Autodesk Inventor part; units mm, degrees
ref_plane "YZ Plane" through (0, 0, 0) normal (1, 0, 0) x (0, 1, 0)
ref_plane "XZ Plane" through (0, 0, 0) normal (0, 1, 0) x (-1, 0, 0)
ref_plane "XY Plane" through (0, 0, 0) normal (0, 0, 1) x (1, 0, 0)
sketch "Skizze1" plane through (0, 0, 0) normal (0, 1, 0) x (-1, 0, 0)
  line L0 (0, 0) -> (30, 0)
  line L1 (30, 0) -> (30, 30)
  line L2 (30, 30) -> (0, 30)
  line L3 (0, 30) -> (0, 0)
  circle A0 centre (15, 15) radius 14.1
  dimension "d7" = 28.2
  dimension "d20" = 30
  dimension "d21" = 30
extrude "Extrusion1" add sketch "Skizze1" along normal blind 22 contours L3 L2 L1 L0 | A0
sketch "Skizze2" plane through (0, 22, 0) normal (0, 1, 0) x (1, 0, 0)
  line L0 (0, 0) -> (-30, 0)
  line L1 (-1.5, 0) -> (-28.5, 0)
  line L2 (-28.5, 0) -> (-28.5, -28.5)
  line L3 (-28.5, -28.5) -> (-1.5, -28.5)
  line L4 (-1.5, -28.5) -> (-1.5, 0)
  line L5 (-30, 0) -> (-30, -30)
  line L6 (0, -30) -> (0, 0)
  line L7 (-30, -30) -> (0, -30)
  dimension "d8" = 1.5
  dimension "d9" = 1.5
  dimension "d10" = 1.5
extrude "Extrusion2" cut sketch "Skizze2" against normal blind 22 contours L4 L3 L2 L0
sketch "Skizze5" plane through (0, 22, 0) normal (0, 1, 0) x (1, 0, 0)
  line L0 (-30, 0) -> (-30, -30)
  line L1 (0, 0) -> (-30, 0)
  line L2 (-30, 0) -> (-30, -30)
  line L3 (-30, -30) -> (0, -30)
  line L4 (0, -30) -> (0, 0)
  line L5 (-31.5556, 0) -> (-1.5, 0) construction
  circle A0 centre (-15, -15) radius 1.35
  line L6 (-1.5, -28.5) -> (-28.5, -28.5)
  line L7 (-1.5, 0) -> (-1.5, -28.5)
  line L8 (-28.5, -28.5) -> (-28.5, 0)
  line L9 (-1.5, -28.5) -> (-28.5, -28.5)
  dimension "d17" = 2.7
extrude "Extrusion4" add sketch "Skizze5" along normal blind 1.5
equation "\"Biegeradius\" = Stärke"
equation "\"BreiteBiegungsfreistellung\" = Stärke"
equation "\"TiefeBiegungsfreistellung\" = 0.5 * Stärke"
equation "\"GrößeEckenfreistellung\" = 4 * Stärke"
equation "\"MinimalRest\" = 2 * Stärke"
equation "\"Übergangsradius\" = Biegeradius"
equation "\"JacobiRadiusGröße\" = Biegeradius"
equation "\"Abstandsgröße\" = Stärke"
properties part number "Gehäuse Motor"
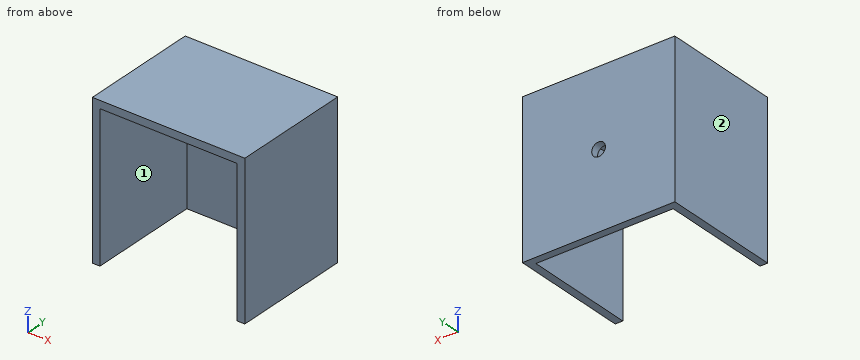
For this review, take the finished solid that the model builds, in its own axes (mm). Face numbers are marked on the shaded views. A direction names the side the tool comes from. Give positions to 0.01 mm unless a question says otherwise; leave off trailing zeros. Loops run counter-clockwise (first coordinate to the right, second up) from the corner with the lowest first, then second, coordinate; pieces in that order, holes last.
Item 1: Take a section at C-C, the plane x = -15.75. State the section outline as (y, z) points.
Item 2: Take a section at D-D, the plane x = -27.25. State the section outline as (y, z) points.
Item 3: Tool access review of the marked faces 1 and 2: name each direction out of +Z, -Z, +X, -X, +Y, -Y from which nothing blocks a thin tool from reaching the whole face with its end or side.
Item 4: Take a section at A-A, the plane z = 15. State the section outline as (x, y) points.
Item 5: Insertion check: pin 1 (2 mm diameter, centred on x = -23.5, z = 11.5, fed in from -Y); pin 2 (11 mm diameter, centred on x = -16, y = 8.5, fed in from -Z). Each pin has a flat end and moves straight along its axis. Give the tip position at first contact, or say it passes through.
Item 6: Take a section at B-B, the plane y = 3.75. State the section outline as (x, z) points.
Item 7: For line 1 along X through (y, z) = (22.6, 15); line 2 along X through (y, z) = (6.75, 14); line 3 along Z through (x, y) = (-15, 22.4), list the stretches that pass through material, from the lowest coordinate up.
Calculated:
1. outline: (0, 28.5) - (22, 28.5) - (22, 16.12) - (23.5, 16.12) - (23.5, 30) - (0, 30) - close; (22, 0) - (23.5, 0) - (23.5, 13.88) - (22, 13.88) - close
2. outline: (0, 28.5) - (22, 28.5) - (22, 0) - (23.5, 0) - (23.5, 30) - (0, 30) - close
3. face 1: -Z, -Y
3. face 2: +Z, -Z, -X, +Y, -Y
4. outline: (-30, 0) - (-28.5, 0) - (-28.5, 22) - (-16.35, 22) - (-16.35, 23.5) - (-30, 23.5) - close; (-13.65, 22) - (-1.5, 22) - (-1.5, 0) - (0, 0) - (0, 23.5) - (-13.65, 23.5) - close
5. pin 1: stops at y = 22
5. pin 2: stops at z = 28.5
6. outline: (-30, 0) - (-28.5, 0) - (-28.5, 28.5) - (-1.5, 28.5) - (-1.5, 0) - (0, 0) - (0, 30) - (-30, 30) - close
7. line 1: x = -30 to -16.35, -13.65 to 0
7. line 2: x = -30 to -28.5, -1.5 to 0
7. line 3: z = 0 to 13.65, 16.35 to 30
